Build history of the part. All positions in model axes, mm. Face numbers are marked on the shaded views. A direction names the side the tool comes from. Coordinates: 2 decimals unless noted, no trailing zeros. Write each loop counter-clockwise with the first axis right and the second up, starting at its lowest first coordinate (ties: lowest second). Pieces come first, ordered by that corner, then holes.
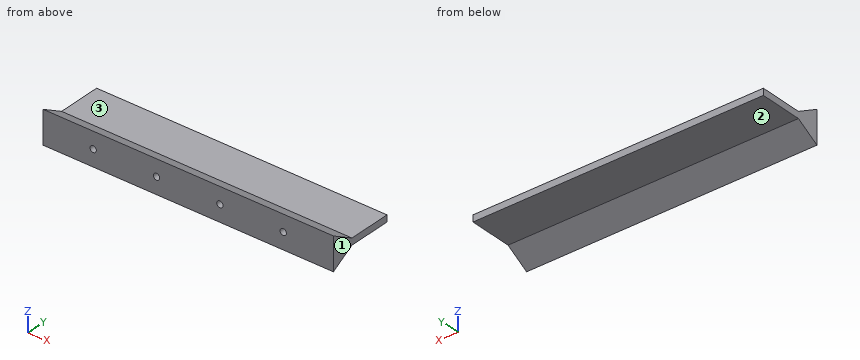
Autodesk Inventor part; units mm, degrees
ref_plane "YZ Plane" through (0, 0, 0) normal (1, 0, 0) x (0, 1, 0)
ref_plane "XZ Plane" through (0, 0, 0) normal (0, 1, 0) x (-1, 0, 0)
ref_plane "XY Plane" through (0, 0, 0) normal (0, 0, 1) x (1, 0, 0)
sketch "Sketch1" plane through (0, 0, 0) normal (0, 0, 1) x (1, 0, 0)
  line L0 (0, 0) -> (220, 0)
  line L1 (220, 0) -> (220, 50)
  line L2 (220, 50) -> (0, 50)
  line L3 (0, 50) -> (0, 0)
  dimension "d0" = 220
  dimension "d1" = 50
extrude "Extrusion1" add sketch "Sketch1" along normal blind 5
sketch "Sketch2" plane through (0, 0, 0) normal (0, -1, 0) x (1, 0, 0)
  line L0 (0, 0) -> (220, 0)
  line L1 (0, 5) -> (220, 5)
  line L2 (0, 0) -> (0, 5)
  point P0 (38, 2.5)
  point P1 (86, 2.5)
  point P2 (134, 2.5)
  point P3 (182, 2.5)
  point P4 (0, 2.5)
  dimension "d4" = 5
  dimension "d5" = 220
  dimension "d6" = 2.5
  dimension "d7" = 38
  dimension "d8" = 48
  dimension "d9" = 48
  dimension "d10" = 48
hole "Hole1" at (38, 0, 2.5) at (86, 0, 2.5) at (134, 0, 2.5) at (182, 0, 2.5) direction (0, 1, 0) diameter 4.8 depth 10
sketch "Sketch3" plane through (0, 0, 0) normal (-1, 0, 0) x (0, 0, 1)
  line L0 (4.9, 0) -> (0.1, 0)
  line L1 (0.1, 10) -> (4.9, 10)
  line L2 (4.9, 0) -> (0.1, 0)
  line L3 (0.1, 10) -> (4.9, 10)
  line L4 (0, 0) -> (-10, 0)
  line L5 (-10, 0) -> (0, 17.3205)
  line L6 (0, 50) -> (0, 0)
  line L7 (5, 50) -> (5, 0)
  line L8 (5, 0) -> (15, 0)
  line L9 (15, 0) -> (5, 17.3205)
  point P0 (66.5733, 11.83)
  dimension "d18" = 10
  dimension "d19" = 60
extrude "Extrusion2" add sketch "Sketch3" against normal up to surface (220 mm away)
properties part number "Disk_Barrier_3DPrint"
1. Saw through at B-B on x = 18. List the corners of the cut face in (y, z).
Computed values:
outline: (0, -10) - (17.32, 0) - (50, 0) - (50, 5) - (17.32, 5) - (0, 15) - close
2. 3-axis set-ups, long thin cutter, end or side, ignore diameter. For the marked faces 1, 2 and 3: which of +Z, -Z, +X, -X, +Y, -Y reach the whole face in a straight line?
Computed values:
face 1: +Z, -Z, +X, +Y, -Y
face 2: -Z, +X, -X, +Y
face 3: +Z, +X, -X, +Y
3. Saw through at C-C on y = 6. List the corners of the cut face in (x, z).
Computed values:
outline: (0, -6.54) - (220, -6.54) - (220, 11.54) - (0, 11.54) - close; hole circle Ø4.8 at (38, 2.5); hole circle Ø4.8 at (86, 2.5); hole circle Ø4.8 at (134, 2.5); hole circle Ø4.8 at (182, 2.5)
4. Saw through at A-A on z = 2.5. List the corners of the cut face in (x, y).
Computed values:
outline: (0, 0) - (35.6, 0) - (35.6, 10) - (40.4, 10) - (40.4, 0) - (83.6, 0) - (83.6, 10) - (88.4, 10) - (88.4, 0) - (131.6, 0) - (131.6, 10) - (136.4, 10) - (136.4, 0) - (179.6, 0) - (179.6, 10) - (184.4, 10) - (184.4, 0) - (220, 0) - (220, 50) - (0, 50) - close
5. Saw through at D-D on y = 28.5. List the corners of the cut face in (x, z), plus the area to 3 significant figures.
Computed values:
outline: (0, 0) - (220, 0) - (220, 5) - (0, 5) - close
area: 1,100 mm2
6. Probe line 1 along X through (y, z) = (5, 2.5); line 2 along Z through (x, y) = (27, 23); line 3 along Z through (x, y) = (38, 6). List the from-to ranges inside material, lowest first.
Computed values:
line 1: x = 0 to 35.6, 40.4 to 83.6, 88.4 to 131.6, 136.4 to 179.6, 184.4 to 220
line 2: z = 0 to 5
line 3: z = -6.54 to 0.1, 4.9 to 11.54
7. Flat gauge pins, fed straight in: pin 1 (16.5 mm diameter, centred on x = 118.5, y = 28, fed in from +Z); pin 2 (1.4 mm diameter, centred on x = 181, z = 1.5, fed in from -Y); pin 3 (3 mm diameter, centred on x = 91, z = -2, fed in from -Y); pin 4 (3 mm diameter, centred on x = 129.5, y = 39, fed in from -Z). Where does each tip first touch, or does it go through?
Computed values:
pin 1: stops at z = 5
pin 2: stops at y = 10
pin 3: stops at y = 0
pin 4: stops at z = 0
